Check sheet for the modelled part. Datum: model origin and axes. Units: mm. Give positions to 0.01 mm unless a question says otherwise; leave off trailing zeros. Loops run counter-clockwise (first coordinate to the right, second up) from the corner with the lowest first, then second, coordinate; pieces in that order, holes last. Notation, with made-up numbers: M 35,0 L 61,0 A9 cw 61,9 Z; hole C 37,80 d2. An arc over 180 degrees is marked long. Put each result on its own line as item: value. Start each with the question number.
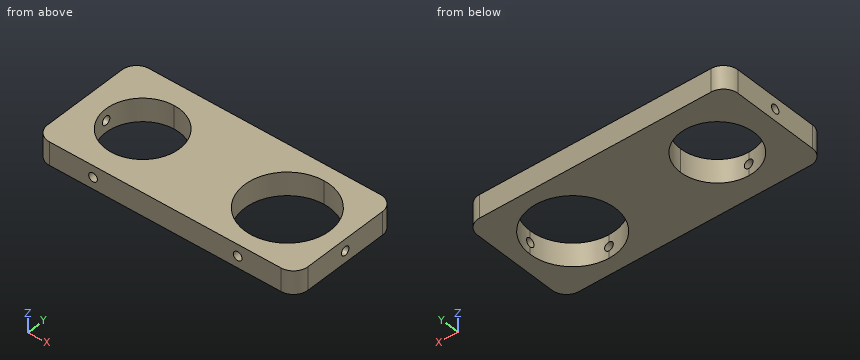
```python
from build123d import *

# Parameters (mm, degrees)
F1_DEPTH = 8
F2_R     = 1.5
F3_DEPTH = 25
F4_R     = 1.5
F5_DEPTH = 25
F6_START = 54.3
F6_DEPTH = 27.9
F7_R     = 5


with BuildPart() as f1:
    # F0 (on Top) → F1 (new body)
    with BuildSketch(Plane.XY):
        with BuildLine():
            ThreePointArc((0, 12.7), (8.9802561211, 8.9802561211), (12.7, 0))
            ThreePointArc((12.7, 0), (8.9802561211, -8.9802561211), (0, -12.7))
            Line((0, -12.7), (0, -20))
            Line((0, -20), (50, -20))
            Line((50, -20), (50, -14.7))
            ThreePointArc((50, -14.7), (35.3, 0), (50, 14.7))
            Line((50, 14.7), (50, 20))
            Line((50, 20), (0, 20))
            Line((0, 20), (0, 12.7))
        make_face()
        with BuildLine():
            ThreePointArc((0, -12.7), (-12.7, 0), (0, 12.7))
            Line((0, 12.7), (0, 20))
            Line((0, 20), (-20, 20))
            Line((-20, 20), (-20, -20))
            Line((-20, -20), (0, -20))
            Line((0, -20), (0, -12.7))
        make_face()
        with BuildLine():
            Line((70, 20), (50, 20))
            Line((50, 20), (50, 14.7))
            ThreePointArc((50, 14.7), (60.3944696834, 10.3944696834), (64.7, 0))
            ThreePointArc((64.7, 0), (60.3944696834, -10.3944696834), (50, -14.7))
            Line((50, -14.7), (50, -20))
            Line((50, -20), (70, -20))
            Line((70, -20), (70, 20))
        make_face()
    extrude(amount=F1_DEPTH)

    # F2 (on Front) → F3 (cut)
    with BuildSketch(Plane.XZ):
        with Locations((0, 4)):
            Circle(F2_R)
        with Locations((50, 4)):
            Circle(F2_R)
    extrude(amount=F3_DEPTH, mode=Mode.SUBTRACT)

    # F4 (on Right) → F5 (cut)
    with BuildSketch(Plane.YZ):
        with Locations((0, 4)):
            Circle(F4_R)
    extrude(amount=-F5_DEPTH, mode=Mode.SUBTRACT)

    # F4 (on Right) → F6 (cut)
    with BuildSketch(Plane.YZ.offset(F6_START)):
        with Locations((0, 4)):
            Circle(F4_R)
    extrude(amount=F6_DEPTH, mode=Mode.SUBTRACT)

    # F7
    f7_edges = [f1.edges().sort_by_distance(p)[0] for p in [
        (70, 20, 4),
        (70, -20, 4),
        (-20, 20, 4),
        (-20, -20, 4),
    ]]
    fillet(f7_edges, radius=F7_R)


solid = f1.part
```
Q1. Thickness scan on line 1 along Z through (x, y) = (67.9, 0); line 2 along X through (y, z) = (-15.75, 4); line 3 along X through (y, z) = (-17.75, 4). Record the ranges inside material, lowest first. Write a range as [from, to].
Q2. Section check A-A, the plane z = 4. Record the cut outline in (x, y), then the cut area to 3 significant figures.
Q3. Section check D-D, the plane x = 11.5. Record the cut outline in (y, z).
Q4. Section check B-B, the plane y = 8. Record the cut outline in (x, z), then the cut area to 3 significant figures.
Q5. Section check C-C, the plane x = -8. Record the cut outline in (y, z).
Q6. Depth check by flat-ended pin: P1, Ø2.5, axis at y = 0, z = 4, coming from the +X side. Enter the tip coordinate at first touch or a pass-through.
Found:
1. line 1: z = [0, 2.5], [5.5, 8]
1. line 2: x = [-19.94, -1.5], [1.5, 48.5], [51.5, 69.94]
1. line 3: x = [-19.18, -1.5], [1.5, 48.5], [51.5, 69.18]
2. outline: M -20,-15 A5 ccw -15,-20 L -1.5,-20 L -1.5,-12.61 A12.7 cw -12.61,-1.5 L -20,-1.5 Z; M -20,1.5 L -12.61,1.5 A12.7 cw long 1.5,-12.61 L 1.5,-20 L 48.5,-20 L 48.5,-14.62 A14.7 cw long 64.62,1.5 L 70,1.5 L 70,15 A5 ccw 65,20 L -15,20 A5 ccw -20,15 Z; M 51.5,-20 L 65,-20 A5 ccw 70,-15 L 70,-1.5 L 64.62,-1.5 A14.7 cw 51.5,-14.62 Z
2. area: 2,320 mm^2
3. outline: M -20,0 L -5.39,0 L -5.39,8 L -20,8 Z; M 5.39,0 L 20,0 L 20,8 L 5.39,8 Z
4. outline: M -20,0 L -9.86,0 L -9.86,8 L -20,8 Z; M 9.86,0 L 37.67,0 L 37.67,8 L 9.86,8 Z; M 62.33,0 L 70,0 L 70,8 L 62.33,8 Z
4. area: 365 mm^2
5. outline: M -20,0 L -9.86,0 L -9.86,8 L -20,8 Z; M 9.86,0 L 20,0 L 20,8 L 9.86,8 Z
6. P1: stops at x = 35.35
